from build123d import *

# Parameters (mm, degrees)
SKETCH1_W             = 60
SKETCH1_H             = 1000
BOSS_EXTRUDE1_DEPTH   = 20
BOSS_EXTRUDE1_2_DEPTH = 20
BOSS_EXTRUDE1_3_DEPTH = 20
BOSS_EXTRUDE1_4_DEPTH = 20
SKETCH2_W             = 1000
SKETCH2_H             = 60
BOSS_EXTRUDE2_DEPTH   = 20
SKETCH3_W             = 85
SKETCH3_H             = 60
BOSS_EXTRUDE3_DEPTH   = 80
SKETCH4_W             = 1000
SKETCH4_H             = 60
BOSS_EXTRUDE4_DEPTH   = 20
SKETCH5_W             = 60
SKETCH5_H             = 1000
BOSS_EXTRUDE5_DEPTH   = 20
SKETCH6_W             = 410
SKETCH6_H             = 20
CUT_EXTRUDE1_DEPTH    = 1000


with BuildPart() as part:
    # Sketch1 → Boss-Extrude1 (new body)
    with BuildSketch(Plane(origin=(0, 0, 0), x_dir=(1, 0, 0), z_dir=(0, 1, 0))):
        with Locations((-470, 0)):
            Rectangle(SKETCH1_W, SKETCH1_H)
    extrude(amount=BOSS_EXTRUDE1_DEPTH)



with BuildPart() as body_2:
    # Sketch1 → Boss-Extrude1 2 (new body)
    with BuildSketch(Plane(origin=(0, 0, 0), x_dir=(1, 0, 0), z_dir=(0, 1, 0))):
        with Locations((470, 0)):
            Rectangle(SKETCH1_W, SKETCH1_H)
    extrude(amount=BOSS_EXTRUDE1_2_DEPTH)


with BuildPart() as body_3:
    # Sketch1 → Boss-Extrude1 3 (new body)
    with BuildSketch(Plane(origin=(0, 0, 0), x_dir=(1, 0, 0), z_dir=(0, 1, 0))):
        with Locations((-156.67, 0)):
            Rectangle(SKETCH1_W, SKETCH1_H)
    extrude(amount=BOSS_EXTRUDE1_3_DEPTH)


with BuildPart() as body_4:
    # Sketch1 → Boss-Extrude1 4 (new body)
    with BuildSketch(Plane(origin=(0, 0, 0), x_dir=(1, 0, 0), z_dir=(0, 1, 0))):
        with Locations((156.67, 0)):
            Rectangle(SKETCH1_W, SKETCH1_H)
    extrude(amount=BOSS_EXTRUDE1_4_DEPTH)


with BuildPart() as part_1:
    add(part.part)

    add(body_2.part)  # Boss-Extrude2 merges body 2

    add(body_3.part)  # Boss-Extrude2 merges body 3

    add(body_4.part)  # Boss-Extrude2 merges body 4
    # Sketch2 → Boss-Extrude2 (add)
    with BuildSketch(Plane(origin=(0, 0, 0), x_dir=(1, 0, 0), z_dir=(0, 1, 0))):
        with Locations((0, -470)):
            Rectangle(SKETCH2_W, SKETCH2_H)
        with Locations((0, 470)):
            Rectangle(SKETCH2_W, SKETCH2_H)
        Rectangle(SKETCH2_W, SKETCH2_H)
    extrude(amount=BOSS_EXTRUDE2_DEPTH)

    # Sketch3 → Boss-Extrude3 (add)
    with BuildSketch(Plane(origin=(0, 20, 0), x_dir=(1, 0, 0), z_dir=(0, 1, 0))):
        with Locations((457.5, -470)):
            Rectangle(SKETCH3_W, SKETCH3_H)
        with Locations((457.5, 470)):
            Rectangle(SKETCH3_W, SKETCH3_H)
        with Locations((457.5, 0)):
            Rectangle(SKETCH3_W, SKETCH3_H)
        with Locations((154.5, -470)):
            Rectangle(SKETCH3_W, SKETCH3_H)
        with Locations((154.5, 0)):
            Rectangle(SKETCH3_W, SKETCH3_H)
        with Locations((154.5, 470)):
            Rectangle(SKETCH3_W, SKETCH3_H)
        with Locations((-154.5, 470)):
            Rectangle(SKETCH3_W, SKETCH3_H)
        with Locations((-154.5, 0)):
            Rectangle(SKETCH3_W, SKETCH3_H)
        with Locations((-154.5, -470)):
            Rectangle(SKETCH3_W, SKETCH3_H)
        with Locations((-457.5, 0)):
            Rectangle(SKETCH3_W, SKETCH3_H)
        with Locations((-457.5, 470)):
            Rectangle(SKETCH3_W, SKETCH3_H)
        with Locations((-457.5, -470)):
            Rectangle(SKETCH3_W, SKETCH3_H)
    extrude(amount=BOSS_EXTRUDE3_DEPTH)

    # Sketch4 → Boss-Extrude4 (add)
    with BuildSketch(Plane(origin=(0, 100, 0), x_dir=(1, 0, 0), z_dir=(0, 1, 0))):
        with Locations((0, -470)):
            Rectangle(SKETCH4_W, SKETCH4_H)
        Rectangle(SKETCH4_W, SKETCH4_H)
        with Locations((0, 470)):
            Rectangle(SKETCH4_W, SKETCH4_H)
    extrude(amount=BOSS_EXTRUDE4_DEPTH)

    # Sketch5 → Boss-Extrude5 (add)
    with BuildSketch(Plane(origin=(0, 120, 0), x_dir=(1, 0, 0), z_dir=(0, 1, 0))):
        with Locations((-470, 0)):
            Rectangle(SKETCH5_W, SKETCH5_H)
        with Locations((-352.5, 0)):
            Rectangle(SKETCH5_W, SKETCH5_H)
        with Locations((-235, 0)):
            Rectangle(SKETCH5_W, SKETCH5_H)
        with Locations((-117.5, 0)):
            Rectangle(SKETCH5_W, SKETCH5_H)
        Rectangle(SKETCH5_W, SKETCH5_H)
        with Locations((117.5, 0)):
            Rectangle(SKETCH5_W, SKETCH5_H)
        with Locations((235, 0)):
            Rectangle(SKETCH5_W, SKETCH5_H)
        with Locations((352.5, 0)):
            Rectangle(SKETCH5_W, SKETCH5_H)
        with Locations((470, 0)):
            Rectangle(SKETCH5_W, SKETCH5_H)
    extrude(amount=-BOSS_EXTRUDE5_DEPTH)

    # Sketch6 → Cut-Extrude1 (cut)
    with BuildSketch(Plane(origin=(500, 0, 0), x_dir=(0, 0, -1), z_dir=(1, 0, 0))):
        with Locations((-235, 10)):
            Rectangle(SKETCH6_W, SKETCH6_H)
        with Locations((235, 10)):
            Rectangle(SKETCH6_W, SKETCH6_H)
    extrude(amount=-CUT_EXTRUDE1_DEPTH, mode=Mode.SUBTRACT)


solid = part_1.part
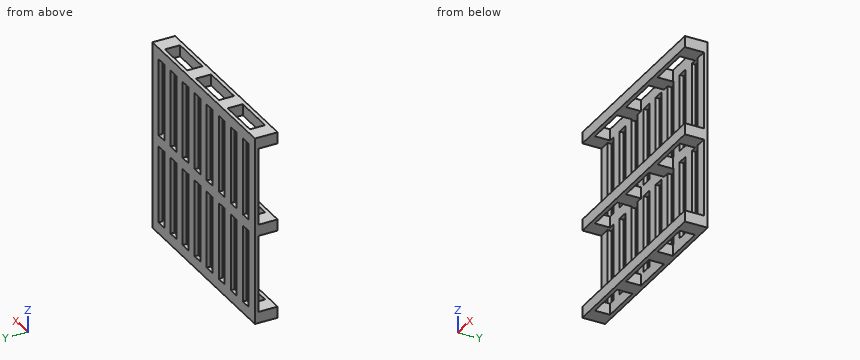
Design review of the part built by this model. Coordinates are the model's own, in mm. Coordinates: 2 decimals unless noted, no trailing zeros. Order: outer loops, then holes, each group sorted by start corner. A loop starts at its lowest first (then second) coordinate and runs counter-clockwise, first axis right, second up. Notation, with made-up numbers: M 72.5,3 L 106.5,3 A21 ccw 106.5,40 Z; hole C 79.25,-22.75 d8. An arc over 180 degrees is marked long. Use a Markdown table: item, result.
(1) Wall thickness on probe 1 along Z at (x, y) = (-172.5, 66.5); probe 2 along X at (y, z) = (78.5, -7); probe 3 along Y at (x, z) = (-217.5, -284): over which ranges is each line inside the solid? List them lowest first.
Worked answers:
| item | result |
|---|---|
| probe 1 | z = -500 to -440, -30 to 30, 440 to 500 |
| probe 2 | x = -500 to -415, -197 to -112, 112 to 197, 415 to 500 |
| probe 3 | y = 100 to 120 |
(2) Add section B-B (y = 61.5). Count the separate pieces of the cut face and the enclosed holes in it, then the cut area to 3 significant figures.
Worked answers:
| item | result |
|---|---|
| separate pieces | 12 |
| enclosed holes | 0 |
| area | 61,200 mm2 |
(3) For P1, Ø4, axis at x = -347.5, z = -202, coming from the -Y side, flat-tipped, find the tip position at first contact; note if it passes through.
Worked answers:
| item | result |
|---|---|
| P1 | stops at y = 100 |
(4) Add section A-A (x = -365). Give the boundary of the cut face in (y, z), then the cut area to 3 significant figures.
Worked answers:
| item | result |
|---|---|
| outline | M 0,-500 L 20,-500 L 20,-440 L 0,-440 Z; M 0,-30 L 20,-30 L 20,30 L 0,30 Z; M 0,440 L 20,440 L 20,500 L 0,500 Z; M 100,-500 L 120,-500 L 120,500 L 100,500 Z |
| area | 23,600 mm2 |
